Source: CAD feature listing. Evaluate the final solid. Frame: model axes, mm. A direction names the side the tool comes from. Coordinates: 2 decimals unless noted, no trailing zeros. Write each loop counter-clockwise with the first axis right and the second up, starting at its lowest first coordinate (ties: lowest second). Pieces come first, ordered by that corner, then holes. Notation, with made-up numbers: M 30,85.25 L 35,85.25 A6 cw 35,91.25 Z; hole C 5,83 d9. An arc over 180 degrees is marked long. One line per item, written item: value. Start each with the question number.
Item 1: Pin query (flat end, axial travel): P1, Ø2.5, axis at x = 57.29, z = -4.83, coming from the +Y side; P2, Ø1.6, axis at y = -1, z = 54, coming from the -X side (3 decimals); P3, Ø1, axis at x = 14.5, y = 17, coming from the +Z side; P4, Ø0.6, axis at x = 47.5, y = 23.5, coming from the +Z side. Return the tip coordinate at first contact, or that it passes through.
Item 2: Cut plane B-B, the plane y = 11.5. Output: boundary loops of the cut face in (x, z), then the cut area to 3 significant figures.
Item 3: Mould query, pull axis X, two halves, no side actions, for faces 1 (the flat face through (7, 23, -6)), 2 (the flat face through (46, 0, 23)), 3 (the cylindrical face through (69.7, 13.02, -32.01)). Classes: released by +X, released by -X, zero draft, split by the parting line, or undercut.
Item 4: Ray query, L1, parallel to Y at x = 41, z = -25; L2, parallel to X at y = 23.75, z = -4.83; L3, parallel to X at y = -0.85, z = -4.83. Return the intervals inside material, ascending. Write a range as from..to.
Item 5: Cut plane C-C, the plane x = 29.5. Output: boundary loops of the cut face in (y, z), then the cut area to 3 significant figures.
Item 6: Set-up query: faces 4 (the flat face through (38, 22.5, -15)), 5 (the flat face through (69.51, 23.49, -6.42)). Return all of +Z, -Z, +X, -X, +Y, -Y with unobstructed straight access to the full face (end or side cutting, diameter ignored); none if empty.
Item 7: Cut plane A-A, the plane z = 67. Output: boundary loops of the cut face in (x, y) (3 decimals), then the cut area to 3 significant figures.
Item 8: Cut plane D-D, the plane x = 9. Output: boundary loops of the cut face in (y, z), then the cut area to 3 significant figures.
```python
from build123d import *

# Parameters (mm, degrees)
BASE_FLANGE1_DEPTH  = 76.09
SKETCH6_W           = 22
SKETCH6_H           = 2
BOSS_EXTRUDE1_DEPTH = 105
FILLET2_R           = 3
CHAMFER1_SIZE       = 13
CHAMFER2_SIZE       = 13
FILLET3_R           = 3
CUT_EXTRUDE1_REACH  = 134.352
CUT_EXTRUDE2_REACH  = 134.352
SKETCH7_3_R         = 1.5
CUT_EXTRUDE3_REACH  = 161.48
SKETCH8_R           = 2.25


# Sheet-metal steps are written as plain solids
with BuildPart() as part:
    # Sketch1 → Base-Flange1 (new body)
    with BuildSketch(Plane(origin=(0, 0, 0), x_dir=(0, 0, -1), z_dir=(1, 0, 0))):
        with BuildLine():
            Line((0, 0), (30.56, 0))
            ThreePointArc((30.56, 0), (30.871126984, 0.128873016), (31, 0.44))
            Line((31, 0.44), (31, 22.06))
            ThreePointArc((31, 22.06), (30.871126984, 22.371126984), (30.56, 22.5))
            Line((30.56, 22.5), (0, 22.5))
            Line((0, 22.5), (0, 24.5))
            Line((0, 24.5), (30.56, 24.5))
            ThreePointArc((30.56, 24.5), (32.285340546, 23.785340546), (33, 22.06))
            Line((33, 22.06), (33, 0.44))
            ThreePointArc((33, 0.44), (32.285340546, -1.285340546), (30.56, -2))
            Line((30.56, -2), (0, -2))
            Line((0, -2), (0, 0))
        make_face()
    extrude(amount=BASE_FLANGE1_DEPTH)

    # Sketch6 → Boss-Extrude1 (add)
    with BuildSketch(Plane.XY):
        with Locations((38.045, -1)):
            Rectangle(SKETCH6_W, SKETCH6_H)
    extrude(amount=BOSS_EXTRUDE1_DEPTH)

    # Fillet2
    fillet2_edges = [part.edges().sort_by_distance(p)[0] for p in [
        (49.045, -1, 0),
        (27.045, -1, 0),
    ]]
    fillet(fillet2_edges, radius=FILLET2_R)

    # Chamfer1
    chamfer1_edges = [part.edges().sort_by_distance(p)[0] for p in [
        (0, -1, 0),
        (0, 23.5, 0),
    ]]
    chamfer(chamfer1_edges, length=CHAMFER1_SIZE)

    # Chamfer2
    chamfer2_edges = [part.edges().sort_by_distance(p)[0] for p in [
        (76.09, -1, 0),
        (76.09, 23.5, 0),
    ]]
    chamfer(chamfer2_edges, length=CHAMFER2_SIZE)

    # Fillet3
    fillet3_edges = [part.edges().sort_by_distance(p)[0] for p in [
        (76.09, -1, -13),
        (76.09, 23.5, -13),
        (63.09, -1, 0),
        (63.09, 23.5, 0),
        (13, 23.5, 0),
        (13, -1, 0),
        (0, -1, -13),
        (0, 23.5, -13),
    ]]
    fillet(fillet3_edges, radius=FILLET3_R)

    # Sketch7 → Cut-Extrude1 (cut, up to next)
    with BuildSketch(Plane.XZ.offset(2), mode=Mode.PRIVATE) as cut_extrude1_sk1:
        with BuildLine():
            Line((39.995, -18.56), (39.995, -12.56))
            ThreePointArc((39.995, -12.56), (38.045, -10.61), (36.095, -12.56))
            Line((36.095, -12.56), (36.095, -18.56))
            ThreePointArc((36.095, -18.56), (38.045, -20.51), (39.995, -18.56))
        make_face()
    cut_extrude1_tool1 = extrude(cut_extrude1_sk1.sketch, amount=-CUT_EXTRUDE1_REACH, mode=Mode.PRIVATE) & part.part
    # Sketch7 → Cut-Extrude1 (cut, up to next)
    with BuildSketch(Plane.XZ.offset(2), mode=Mode.PRIVATE) as cut_extrude1_sk2:
        with BuildLine():
            Line((39.995, -4.56), (39.995, 1.44))
            ThreePointArc((39.995, 1.44), (38.045, 3.39), (36.095, 1.44))
            Line((36.095, 1.44), (36.095, -4.56))
            ThreePointArc((36.095, -4.56), (38.045, -6.51), (39.995, -4.56))
        make_face()
    cut_extrude1_tool2 = extrude(cut_extrude1_sk2.sketch, amount=-CUT_EXTRUDE1_REACH, mode=Mode.PRIVATE) & part.part
    # Sketch7 → Cut-Extrude1 (cut, up to next)
    with BuildSketch(Plane.XZ.offset(2), mode=Mode.PRIVATE) as cut_extrude1_sk3:
        with BuildLine():
            Line((39.995, 9.44), (39.995, 15.44))
            ThreePointArc((39.995, 15.44), (38.045, 17.39), (36.095, 15.44))
            Line((36.095, 15.44), (36.095, 9.44))
            ThreePointArc((36.095, 9.44), (38.045, 7.49), (39.995, 9.44))
        make_face()
    cut_extrude1_tool3 = extrude(cut_extrude1_sk3.sketch, amount=-CUT_EXTRUDE1_REACH, mode=Mode.PRIVATE) & part.part
    # Sketch7 → Cut-Extrude1 (cut, up to next)
    with BuildSketch(Plane.XZ.offset(2), mode=Mode.PRIVATE) as cut_extrude1_sk4:
        with BuildLine():
            Line((39.995, 23.44), (39.995, 29.44))
            ThreePointArc((39.995, 29.44), (38.045, 31.39), (36.095, 29.44))
            Line((36.095, 29.44), (36.095, 23.44))
            ThreePointArc((36.095, 23.44), (38.045, 21.49), (39.995, 23.44))
        make_face()
    cut_extrude1_tool4 = extrude(cut_extrude1_sk4.sketch, amount=-CUT_EXTRUDE1_REACH, mode=Mode.PRIVATE) & part.part
    # Sketch7 → Cut-Extrude1 (cut, up to next)
    with BuildSketch(Plane.XZ.offset(2), mode=Mode.PRIVATE) as cut_extrude1_sk5:
        with BuildLine():
            Line((39.995, 37.44), (39.995, 43.44))
            ThreePointArc((39.995, 43.44), (38.045, 45.39), (36.095, 43.44))
            Line((36.095, 43.44), (36.095, 37.44))
            ThreePointArc((36.095, 37.44), (38.045, 35.49), (39.995, 37.44))
        make_face()
    cut_extrude1_tool5 = extrude(cut_extrude1_sk5.sketch, amount=-CUT_EXTRUDE1_REACH, mode=Mode.PRIVATE) & part.part
    # Sketch7 → Cut-Extrude1 (cut, up to next)
    with BuildSketch(Plane.XZ.offset(2), mode=Mode.PRIVATE) as cut_extrude1_sk6:
        with BuildLine():
            Line((39.995, 51.44), (39.995, 57.44))
            ThreePointArc((39.995, 57.44), (38.045, 59.39), (36.095, 57.44))
            Line((36.095, 57.44), (36.095, 51.44))
            ThreePointArc((36.095, 51.44), (38.045, 49.49), (39.995, 51.44))
        make_face()
    cut_extrude1_tool6 = extrude(cut_extrude1_sk6.sketch, amount=-CUT_EXTRUDE1_REACH, mode=Mode.PRIVATE) & part.part
    # Sketch7 → Cut-Extrude1 (cut, up to next)
    with BuildSketch(Plane.XZ.offset(2), mode=Mode.PRIVATE) as cut_extrude1_sk7:
        with BuildLine():
            Line((39.995, 65.44), (39.995, 71.44))
            ThreePointArc((39.995, 71.44), (38.045, 73.39), (36.095, 71.44))
            Line((36.095, 71.44), (36.095, 65.44))
            ThreePointArc((36.095, 65.44), (38.045, 63.49), (39.995, 65.44))
        make_face()
    cut_extrude1_tool7 = extrude(cut_extrude1_sk7.sketch, amount=-CUT_EXTRUDE1_REACH, mode=Mode.PRIVATE) & part.part
    # Sketch7 → Cut-Extrude1 (cut, up to next)
    with BuildSketch(Plane.XZ.offset(2), mode=Mode.PRIVATE) as cut_extrude1_sk8:
        with BuildLine():
            Line((39.995, 79.44), (39.995, 85.44))
            ThreePointArc((39.995, 85.44), (38.045, 87.39), (36.095, 85.44))
            Line((36.095, 85.44), (36.095, 79.44))
            ThreePointArc((36.095, 79.44), (38.045, 77.49), (39.995, 79.44))
        make_face()
    cut_extrude1_tool8 = extrude(cut_extrude1_sk8.sketch, amount=-CUT_EXTRUDE1_REACH, mode=Mode.PRIVATE) & part.part
    # Sketch7 → Cut-Extrude1 (cut, up to next)
    with BuildSketch(Plane.XZ.offset(2), mode=Mode.PRIVATE) as cut_extrude1_sk9:
        with BuildLine():
            Line((39.995, 93.44), (39.995, 99.44))
            ThreePointArc((39.995, 99.44), (38.045, 101.39), (36.095, 99.44))
            Line((36.095, 99.44), (36.095, 93.44))
            ThreePointArc((36.095, 93.44), (38.045, 91.49), (39.995, 93.44))
        make_face()
    cut_extrude1_tool9 = extrude(cut_extrude1_sk9.sketch, amount=-CUT_EXTRUDE1_REACH, mode=Mode.PRIVATE) & part.part
    add(cut_extrude1_tool1.solids().sort_by_distance((38.045, -2, -15.56))[0], mode=Mode.SUBTRACT)
    add(cut_extrude1_tool2.solids().sort_by_distance((38.045, -2, -1.56))[0], mode=Mode.SUBTRACT)
    add(cut_extrude1_tool3.solids().sort_by_distance((38.045, -2, 12.44))[0], mode=Mode.SUBTRACT)
    add(cut_extrude1_tool4.solids().sort_by_distance((38.045, -2, 26.44))[0], mode=Mode.SUBTRACT)
    add(cut_extrude1_tool5.solids().sort_by_distance((38.045, -2, 40.44))[0], mode=Mode.SUBTRACT)
    add(cut_extrude1_tool6.solids().sort_by_distance((38.045, -2, 54.44))[0], mode=Mode.SUBTRACT)
    add(cut_extrude1_tool7.solids().sort_by_distance((38.045, -2, 68.44))[0], mode=Mode.SUBTRACT)
    add(cut_extrude1_tool8.solids().sort_by_distance((38.045, -2, 82.44))[0], mode=Mode.SUBTRACT)
    add(cut_extrude1_tool9.solids().sort_by_distance((38.045, -2, 96.44))[0], mode=Mode.SUBTRACT)

    # Cut-Extrude2: up to this face of the body (flat: up to its plane)
    cut_extrude2_end = Plane(part.part.faces().sort_by_distance((38.045, 24.5, -16.141358018))[0])
    # Sketch7<3> → Cut-Extrude2 (cut, up to the picked face)
    with BuildSketch(Plane.XZ.offset(2), mode=Mode.PRIVATE) as cut_extrude2_sk1:
        with Locations(Location((18.8, -4.83, 0), (0, 0, 270))):
            Circle(SKETCH7_3_R)
    cut_extrude2_tool1 = split(extrude(cut_extrude2_sk1.sketch, amount=-CUT_EXTRUDE2_REACH, mode=Mode.PRIVATE), bisect_by=cut_extrude2_end, keep=Keep.BOTH, mode=Mode.PRIVATE)
    # Sketch7<3> → Cut-Extrude2 (cut, up to the picked face)
    with BuildSketch(Plane.XZ.offset(2), mode=Mode.PRIVATE) as cut_extrude2_sk2:
        with Locations(Location((57.29, -4.83, 0), (0, 0, 270))):
            Circle(SKETCH7_3_R)
    cut_extrude2_tool2 = split(extrude(cut_extrude2_sk2.sketch, amount=-CUT_EXTRUDE2_REACH, mode=Mode.PRIVATE), bisect_by=cut_extrude2_end, keep=Keep.BOTH, mode=Mode.PRIVATE)
    add(cut_extrude2_tool1.solids().sort_by(Axis((18.8, -2, -4.83), (0, 1, 0)))[0], mode=Mode.SUBTRACT)
    add(cut_extrude2_tool2.solids().sort_by(Axis((57.29, -2, -4.83), (0, 1, 0)))[0], mode=Mode.SUBTRACT)

    # Sketch8 → Cut-Extrude3 (cut, up to next)
    with BuildSketch(Plane(origin=(0, 0, -33), x_dir=(-1, 0, 0), z_dir=(0, 0, -1)), mode=Mode.PRIVATE) as cut_extrude3_sk1:
        with Locations((-8.05, 11.5)):
            Circle(SKETCH8_R)
    cut_extrude3_tool1 = extrude(cut_extrude3_sk1.sketch, amount=-CUT_EXTRUDE3_REACH, mode=Mode.PRIVATE) & part.part
    # Sketch8 → Cut-Extrude3 (cut, up to next)
    with BuildSketch(Plane(origin=(0, 0, -33), x_dir=(-1, 0, 0), z_dir=(0, 0, -1)), mode=Mode.PRIVATE) as cut_extrude3_sk2:
        with Locations((-68.04, 11.5)):
            Circle(SKETCH8_R)
    cut_extrude3_tool2 = extrude(cut_extrude3_sk2.sketch, amount=-CUT_EXTRUDE3_REACH, mode=Mode.PRIVATE) & part.part
    add(cut_extrude3_tool1.solids().sort_by_distance((8.05, 11.5, -33))[0], mode=Mode.SUBTRACT)
    add(cut_extrude3_tool2.solids().sort_by_distance((68.04, 11.5, -33))[0], mode=Mode.SUBTRACT)


solid = part.part
```
From the geometry:
1. P1: passes through
1. P2: stops at x = 27.045
1. P3: stops at z = -31
1. P4: stops at z = 0
2. outline: M 0,-33 L 5.8,-33 L 5.8,-31 L 0,-31 Z; M 10.3,-33 L 65.79,-33 L 65.79,-31 L 10.3,-31 Z; M 70.29,-33 L 76.09,-33 L 76.09,-31 L 70.29,-31 Z
2. area: 134 mm²
3. face 1: released by -X
3. face 2: zero draft
3. face 3: undercut
4. L1: y = -2..0, 22.5..24.5
4. L2: x = 8.17..17.3, 20.3..55.79, 58.79..67.92
4. L3: x = 8.17..17.3, 20.3..36.11, 39.98..55.79, 58.79..67.92
5. outline: M -2,-30.56 A2.44 ccw 0.44,-33 L 22.06,-33 A2.44 ccw 24.5,-30.56 L 24.5,0 L 22.5,0 L 22.5,-30.56 A0.44 cw 22.06,-31 L 0.44,-31 A0.44 cw 0,-30.56 L 0,105 L -2,105 Z
5. area: 385 mm²
6. face 4: +Z, +X, -X
6. face 5: +Z, +X, +Y, -Y
7. outline: M 27.045,-2 L 36.095,-2 L 36.095,0 L 27.045,0 Z; M 39.995,-2 L 49.045,-2 L 49.045,0 L 39.995,0 Z
7. area: 36.2 mm²
8. outline: M -2,-30.56 A2.44 ccw 0.44,-33 L 9.46,-33 L 9.46,-31 L 0.44,-31 A0.44 cw 0,-30.56 L 0,-4 L -2,-4 Z; M 13.54,-33 L 22.06,-33 A2.44 ccw 24.5,-30.56 L 24.5,-4 L 22.5,-4 L 22.5,-30.56 A0.44 cw 22.06,-31 L 13.54,-31 Z
8. area: 150 mm²
